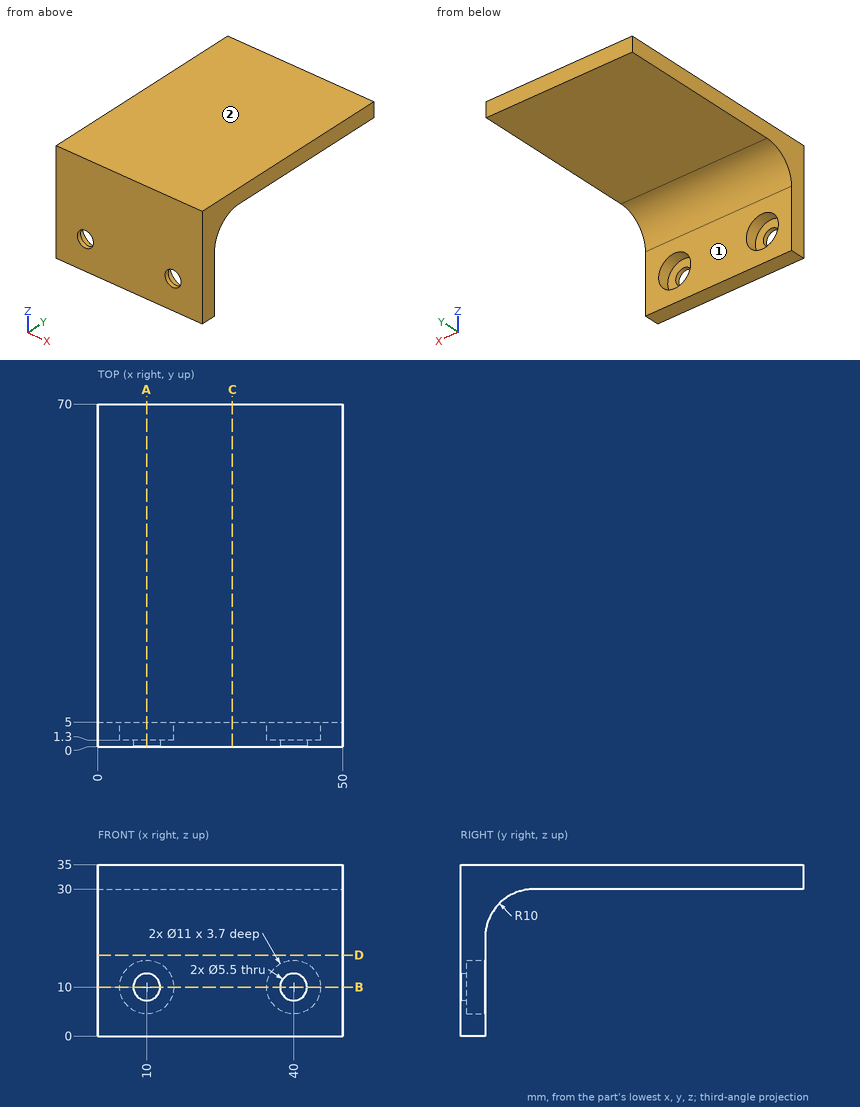
Input: dimensioned drawing with shaded views. Units: mm. Origin: part minimum x, y, z. A direction names the side the tool comes from. Give positions to 0.01 mm unless a question says otherwise; leave off trailing zeros. Order: outer loops, then holes, each group sorted by start corner. A loop starts at its lowest first (then second) coordinate and runs counter-clockwise, first axis right, second up. Notation, with made-up numbers: (20, 22.25) -> (66, 22.25) arc R24 ccw to (66, 59.25) -> close; hole circle Ø11 at (-36, 86). An arc over 180 degrees is marked (long way). Use one line per item in the form item = value.
1) Section C-C, the plane x = 27.5. Return loops of the section in (y, z).
Response values:
outline = (0, 0) -> (5, 0) -> (5, 20) arc R10 cw to (15, 30) -> (70, 30) -> (70, 35) -> (0, 35) -> close
2) Reachability of the marked faces 1 and 2 from +Z, -Z, +X, -X, +Y, -Y: full face, straight path, thin tool, end or side. Return the list, or none.
Response values:
face_1 = -Z, +X, -X, +Y
face_2 = +Z, +X, -X, +Y, -Y
3) Section D-D, the plane z = 16.5. Return loops of the section in (x, y), and give its area (3 significant figures).
Response values:
outline = (0, 0) -> (50, 0) -> (50, 5) -> (0, 5) -> close
area = 250 mm^2
4) Section A-A, the plane x = 10. Return loops of the section in (y, z), and give its area (3 significant figures).
Response values:
outline = (0, 0) -> (5, 0) -> (5, 4.5) -> (1.3, 4.5) -> (1.3, 7.25) -> (0, 7.25) -> close; (0, 12.75) -> (1.3, 12.75) -> (1.3, 15.5) -> (5, 15.5) -> (5, 20) arc R10 cw to (15, 30) -> (70, 30) -> (70, 35) -> (0, 35) -> close
area = 474 mm^2
5) First-contact query: pin 1 Ø3.5 at (x, z) = (8.5, 10) entering from +Y; pin 2 Ø5 at (x, z) = (40, 10) entering from +Y; pin 3 Ø12.5 at (x, z) = (10, 10) entering from +Y; pin 4 Ø25 at (x, y) = (35, 32) entering from -Z. Flat tips, straight axial feed; report the tip coordinate or a pass-through.
Response values:
pin_1 = 1.3
pin_2 = through
pin_3 = 5
pin_4 = 30
6) Section B-B, the plane z = 10. Return loops of the section in (x, y), and give its area (3 significant figures).
Response values:
outline = (0, 0) -> (7.25, 0) -> (7.25, 1.3) -> (4.5, 1.3) -> (4.5, 5) -> (0, 5) -> close; (12.75, 0) -> (37.25, 0) -> (37.25, 1.3) -> (34.5, 1.3) -> (34.5, 5) -> (15.5, 5) -> (15.5, 1.3) -> (12.75, 1.3) -> close; (42.75, 0) -> (50, 0) -> (50, 5) -> (45.5, 5) -> (45.5, 1.3) -> (42.75, 1.3) -> close
area = 154 mm^2
7) Line query: probe 1 along X at (y, z) = (2.65, 10); probe 2 along Z at (x, y) = (10, 1); probe 3 along Z at (x, y) = (6, 23.5). Output: solid intervals per line, ascending.
Response values:
probe_1 = 0 to 4.5, 15.5 to 34.5, 45.5 to 50
probe_2 = 0 to 7.25, 12.75 to 35
probe_3 = 30 to 35
